Check sheet for the drawn part. Datum: minimum x, y, z corner. Units: mm. Coordinates: 2 decimals unless noted, no trailing zeros. Order: outer loops, then holes, each group sorted by start corner. A loop starts at its lowest first (then second) coordinate and runs counter-clockwise, first axis right, second up. Notation, with made-up numbers: (41, 1.5) - (47, 1.5) arc R14 ccw to (47, 28.5) - close; hole circle Ø8 at (55, 62.25). An arc over 180 degrees is marked (long way). Answer as CSV lines item,"result". Start each with the question number.
1. Section check A-A (y = 5). Record the cut outline in (x, z).
2. Section check D-D (z = 26.5). Record the cut outline in (x, y) (1 decimal).
3. Go/stop test with flat-tipped pins: pin 1 (3 mm diameter, centred on x = 2, z = 12.5, fed in from +Y); pin 2 (1 mm diameter, centred on x = 3.5, z = 19.5, fed in from +Y); pin 3 (2.5 mm diameter, centred on y = 32.9, z = 35.84, fed in from -X); pin 4 (3 mm diameter, centred on x = 4.5, z = 5, fed in from +Y). Record where each tip stops, or that it passes through.
4. Material ranges on L1, parallel to Y at x = 1.85, z = 4 (1 decimal); L2, parallel to Z at x = 4, y = 32.5 (1 decimal); L3, parallel to Y at x = 2.4, z = 3 (1 decimal), recorded low to high. Write a range as [from, to].
5. Section check B-B (z = 4). Record the cut outline in (x, y), and give its area (3 significant figures).
6. Section check C-C (x = 0.6). Record the cut outline in (y, z) (1 decimal).
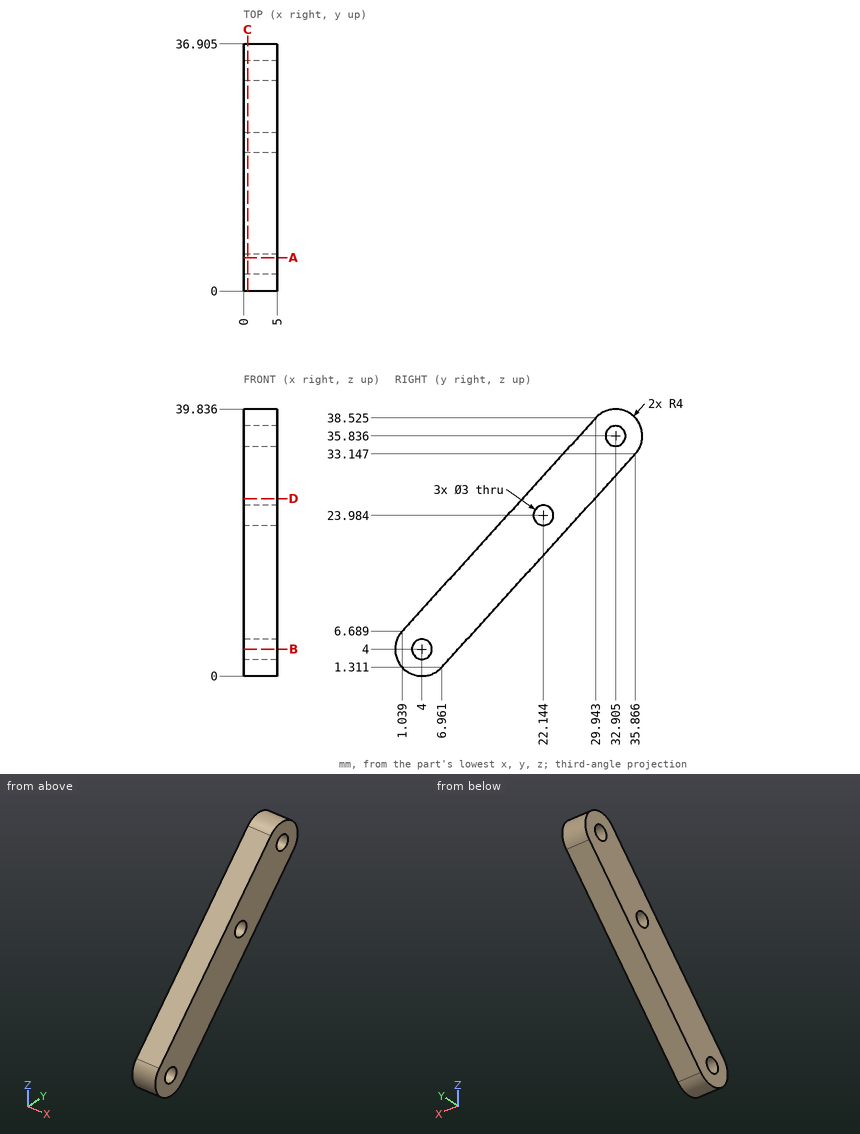
Evaluation:
1,outline,"(0, 0.13) - (5, 0.13) - (5, 2.88) - (0, 2.88) - close; (0, 5.12) - (5, 5.12) - (5, 11.05) - (0, 11.05) - close"
2,outline,"(0, 19) - (5, 19) - (5, 29.8) - (0, 29.8) - close"
3,pin 1,"stops at y = 18.48"
3,pin 2,"stops at y = 23.93"
3,pin 3,"passes through"
3,pin 4,"stops at y = 11.67"
4,L1,"y = [0, 2.5], [5.5, 9.4]"
4,L2,"z = [29.4, 34.4], [37.3, 39.8]"
4,L3,"y = [0.1, 2.9], [5.1, 8.5]"
5,outline,"(0, 0) - (5, 0) - (5, 2.5) - (0, 2.5) - close; (0, 5.5) - (5, 5.5) - (5, 9.4) - (0, 9.4) - close"
5,area,"32.0 mm²"
6,outline,"(1, 6.7) arc R4 ccw to (7, 1.3) - (35.9, 33.1) arc R4 ccw to (29.9, 38.5) - close; hole circle Ø3 at (4, 4); hole circle Ø3 at (22.1, 24); hole circle Ø3 at (32.9, 35.8)"
